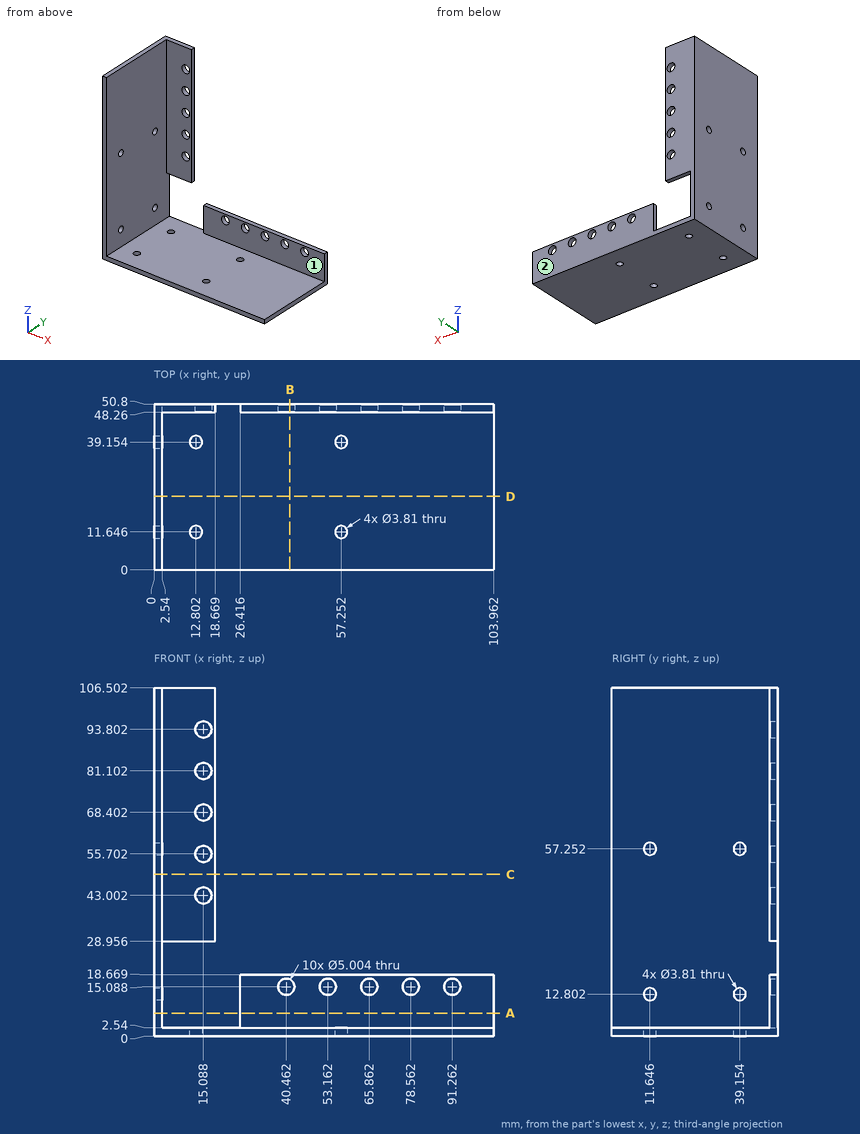
Job drawing, mm, ordinate dimensions from the low corner. One solid piece. A direction names the side the tool comes from. Give positions to 0.01 mm unless a question says otherwise; leave off trailing zeros. Loops run counter-clockwise (first coordinate to the right, second up) from the corner with the lowest first, then second, coordinate; pieces in that order, holes last.
Item 1: Drill centre lines: line 1 (Z direction, x = 40, y = 25); line 2 (Y direction, x = 17.5, z = 57.5). Where is each one in solid material? Low to high.
Answers follow:
line 1: z = 0 to 2.54
line 2: y = 48.26 to 50.8
Item 2: Slice it at C-C, the plane z = 49.5. List the corners of the cut face in (x, y), and give its area (3 significant figures).
Answers follow:
outline: (0, 0) - (2.54, 0) - (2.54, 48.26) - (18.67, 48.26) - (18.67, 50.8) - (0, 50.8) - close
area: 170 mm2
Item 3: Which spindle directions (+Z, -Z, +X, -X, +Y, -Y) get a long thin tool onto all of the face, cutting with end or side? Do the marked faces 1 and 2. Say none if no direction does.
Answers follow:
face 1: +Z, +X, -Y
face 2: +Z, -Z, +X, -X, +Y
Item 4: Slice it at B-B, the plane x = 41.5. List the corners of the cut face in (y, z).
Answers follow:
outline: (0, 0) - (50.8, 0) - (50.8, 12.81) - (48.26, 12.81) - (48.26, 2.54) - (0, 2.54) - close; (48.26, 17.36) - (50.8, 17.36) - (50.8, 18.67) - (48.26, 18.67) - close
Item 5: Slice it at D-D, the plane y = 22.5. List the corners of the cut face in (x, z), and give its area (3 significant figures).
Answers follow:
outline: (0, 0) - (103.96, 0) - (103.96, 2.54) - (2.54, 2.54) - (2.54, 106.5) - (0, 106.5) - close
area: 528 mm2
Item 6: Flat gauge pins, fed straight in: pin 1 (15 mm diameter, centred on x = 68.5, y = 30, fed in from +Z); pin 2 (5 mm diameter, centred on x = 9.5, z = 55, fed in from -Y); pin 3 (1 mm diameter, centred on y = 26, z = 39, fed in from +X). Where does each tip first touch, or does it go through?
Answers follow:
pin 1: stops at z = 2.54
pin 2: stops at y = 48.26
pin 3: stops at x = 2.54
Item 7: Slice it at A-A, the plane z = 7. List the corners of the cut face in (x, y).
Answers follow:
outline: (0, 0) - (2.54, 0) - (2.54, 50.8) - (0, 50.8) - close; (26.42, 48.26) - (103.96, 48.26) - (103.96, 50.8) - (26.42, 50.8) - close
